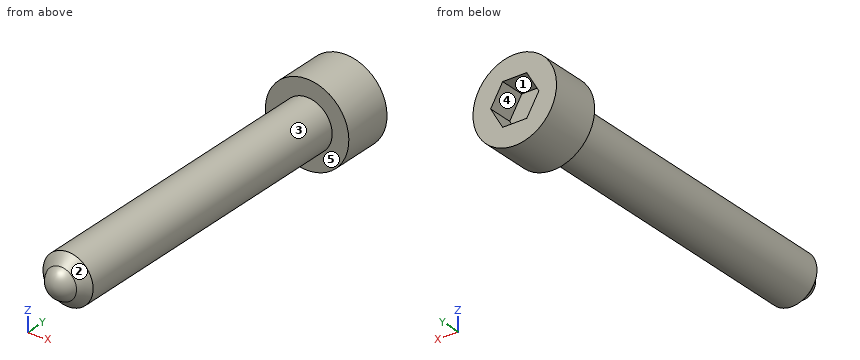
from build123d import *

# Parameters (mm, degrees)
CUT_EXTRUDE1_DEPTH = 3


with BuildPart() as part:
    # Sketch1 → Revolve1 (revolve)
    with BuildSketch(Plane.XY, mode=Mode.PRIVATE) as revolve1_sk:
        with BuildLine():
            Line((3, -37.5734994), (3, 0))
            Line((3, 0), (5, 0))
            Line((5, 0), (5, 6))
            Line((5, 6), (0, 6))
            Line((0, 6), (0, -40))
            ThreePointArc((0, -40), (1.140175425, -39.643167673), (1.8734994, -38.7))
            Line((1.8734994, -38.7), (3, -37.5734994))
        make_face()
    revolve(revolve1_sk.sketch.rotate(Axis((0, 61.691642626, 0), (0, -1, 0)), 90), axis=Axis((0, 61.691642626, 0), (0, -1, 0)))

    # Sketch2 → Cut-Extrude1 (cut)
    with BuildSketch(Plane(origin=(0, 6, 0), x_dir=(-1, 0, 0), z_dir=(0, 1, 0))):
        Polygon((-1.443375673, -2.5), (1.443375673, -2.5), (2.886751346, 0), (1.443375673, 2.5), (-1.443375673, 2.5), (-2.886751346, 0), align=None)
    extrude(amount=-CUT_EXTRUDE1_DEPTH, mode=Mode.SUBTRACT)


solid = part.part
Can you work these out from the model? Positions are in its coordinate system, mm. Face numbers are marked on the shaded views. A direction names the side the tool comes from. Coordinates: 2 decimals unless noted, no trailing zeros. Loops run counter-clockwise (first coordinate to the right, second up) from the corner with the lowest first, then second, coordinate; pieces in that order, holes last. Notation, with made-up numbers: M 22,58.25 L 26,58.25 A19 ccw 26,64.25 Z; hole C 89,-34 d10. An arc over 180 degrees is marked long. Return JSON: item names as keys, results as strings. Group by question number.
Item 1: Imagine slicing it at A-A (y = 3.5). Please give me the cut outline in (x, z), and give its area (3 significant figures).
Item 2: Imagine slicing it at B-B (x = 0). Please give me the cut outline in (y, z), and give its area (3 significant figures).
Item 3: Imagine slicing it at C-C (z = 4). Please give me the cut outline in (x, y).
Item 4: Thinking about a two-plate mould opening in Z: for the marked faces 3, 4 and 5, which applies, released by +Z, released by -Z, zero draft, split by the parting line, or undercut?
Item 5: On a 3-axis mill with a long thin cutter (end or side, diameter ignored), from which of +Z, -Z, +X, -X, +Y, -Y can I reach the whole of each face in a straight line? I mean the marked faces 1 and 2. Say none if no direction works.
Item 6: If I drill on L1, parallel to Y at x = 0.25, z = 3.25; L2, parallel to Z at x = 4, y = 3.5, over which ranges is the centre line in solid material (lowest first)? Write a range as from..to.
Item 7: I'm going to push flat-ended pins straight in: pin 1 Ø6 at (x, y) = (-2, -25) entering from +Z; pin 2 Ø3 at (x, z) = (1.5, 2) entering from -Y; pin 3 Ø5 at (x, y) = (2, -13.5) entering from -Z. Where does each tip first touch, or does it pass through?
Item 8: Imagine slicing it at D-D (y = -19.5). Please give me the cut outline in (x, z), and give its area (3 significant figures).
Verdict:
{
 "1": {"outline": "C 0,0 d10; hole M -2.89,0 L -1.44,-2.5 L 1.44,-2.5 L 2.89,0 L 1.44,2.5 L -1.44,2.5 Z", "area": "56.9 mm^2"},
 "2": {"outline": "M -38.7,-1.87 L -37.57,-3 L 0,-3 L 0,-5 L 6,-5 L 6,-2.5 L 3,-2.5 L 3,2.5 L 6,2.5 L 6,5 L 0,5 L 0,3 L -37.57,3 L -38.7,1.87 A2 ccw Z", "area": "279 mm^2"},
 "3": {"outline": "M -3,0 L 3,0 L 3,6 L -3,6 Z"},
 "4": {"face 3": "split by the parting line", "face 4": "undercut", "face 5": "zero draft"},
 "5": {"face 1": "+Y", "face 2": "-Y"},
 "6": {"L1": "y = 0..6", "L2": "z = -3..3"},
 "7": {"pin 1": "stops at z = 3", "pin 2": "stops at y = -39.73", "pin 3": "stops at z = -3"},
 "8": {"outline": "C 0,0 d6", "area": "28.3 mm^2"}
}
